from build123d import *

# Parameters (mm, degrees)
CUT_EXTRUDE2_DEPTH = 9.0000094


with BuildPart() as part:
    # Sketch1 → Revolve1 (revolve)
    with BuildSketch(Plane(origin=(0, 0, 0), x_dir=(0, 1, 0), z_dir=(0, 0, 1))):
        with BuildLine():
            Line((4.0000047, 0), (-4.0000047, 0))
            Line((-4.0000047, 0), (-4.0000047, 15.200621907))
            ThreePointArc((-4.0000047, 15.200621907), (-3.862299847, 15.545211447), (-3.525035946, 15.699994))
            ThreePointArc((-3.525035946, 15.699994), (-2.891173009, 15.55542644), (-2.425734949, 15.101499778))
            Line((-2.425734949, 15.101499778), (-1.558842609, 13.5999982))
            ThreePointArc((-1.558842609, 13.5999982), (0, 12.7), (1.558842609, 13.5999982))
            Line((1.558842609, 13.5999982), (2.425734949, 15.101499778))
            ThreePointArc((2.425734949, 15.101499778), (2.891173009, 15.55542644), (3.525035946, 15.699994))
            ThreePointArc((3.525035946, 15.699994), (3.862299847, 15.545211447), (4.0000047, 15.200621907))
            Line((4.0000047, 15.200621907), (4.0000047, 0))
        make_face()
    revolve(axis=Axis((0, 4.0000047, 0), (0, -1, 0)))

    # Sketch2 → Cut-Extrude2 (cut, through all)
    with BuildSketch(Plane.XZ.offset(4.0000047)):
        Polygon((7.332348419, 0), (3.666174209, 6.35), (-3.666174209, 6.35), (-7.332348419, 0), (-3.666174209, -6.35), (3.666174209, -6.35), align=None)
    extrude(amount=-CUT_EXTRUDE2_DEPTH, mode=Mode.SUBTRACT)


solid = part.part
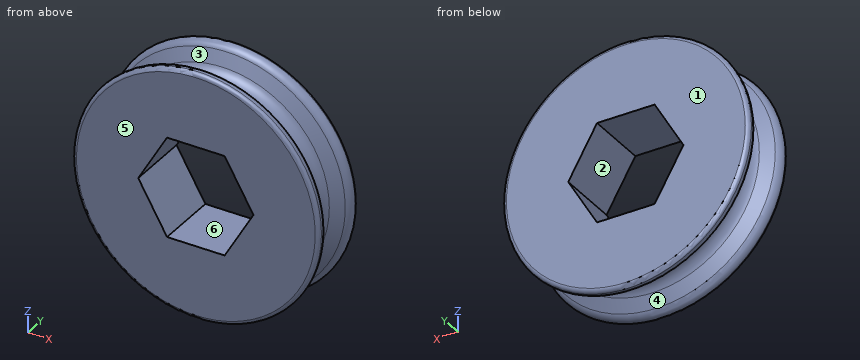
Could you check a few things on this model? Use its own coordinates, in mm. Face numbers are marked on the shaded views. A direction names the side the tool comes from. Coordinates: 2 decimals unless noted, no trailing zeros. Order: outer loops, then holes, each group sorted by start corner. A loop starts at its lowest first (then second) coordinate and runs counter-clockwise, first axis right, second up. Notation, with made-up numbers: (32, 63.25) -> (60, 63.25) arc R10 cw to (60, 82.25) -> close; hole circle Ø8 at (-16, 74). An arc over 180 degrees is marked (long way). One line per item, written item: value. Start each with the question number.
1) If I drill on L1, parallel to X at y = -2.75, z = 0; L2, parallel to Z at x = -1.5, y = 1.75; L3, parallel to Z at x = 6.5, y = -1, over which ranges is the centre line in solid material (lowest first)? Write a range as [from, to].
2) Which directions (+Z, -Z, +X, -X, +Y, -Y) give clear straight access to the entire face, cutting with the end or side of a thin tool? Please do the marked faces 1, 2 and 3.
3) We'd pull the mould along X, two halves only. Please class the marked faces 4, 5 and 6: +X half, -X half, draft (parallel to the pull), parting line (faces both ways), or undercut.
4) I'm going to push flat-ended pins straight in: pin 1 (3 mm diameter, centred on x = -6.5, y = -0.5, fed in from +Z); pin 2 (3 mm diameter, centred on x = 10.5, y = 2, fed in from +Z); pin 3 (1.5 mm diameter, centred on x = 12, y = 2.5, fed in from +Z). Where does each tip first touch, or does it pass through?
5) Imagine slicing it at A-A on x = 0. List the corners of the cut face in (y, z) for me.
Answer list:
1. L1: x = [-15.47, -7.33], [7.33, 15.47]
1. L2: z = [-13.85, -6.35], [6.35, 13.85]
1. L3: z = [-11.26, -1.44], [1.44, 11.26]
2. face 1: +Z, -Z, +X, -X, +Y
2. face 2: +Y, -Y
2. face 3: none
3. face 4: parting line
3. face 5: draft
3. face 6: undercut
4. pin 1: stops at z = 12.9
4. pin 2: stops at z = 12.48
4. pin 3: stops at z = 10.63
5. outline: (-4, -15.2) arc R0.5 ccw to (-3.53, -15.7) arc R1.2 ccw to (-2.43, -15.1) -> (-1.56, -13.6) arc R1.8 cw to (1.56, -13.6) -> (2.43, -15.1) arc R1.2 ccw to (3.53, -15.7) arc R0.5 ccw to (4, -15.2) -> (4, -6.35) -> (-4, -6.35) -> close; (-4, 6.35) -> (4, 6.35) -> (4, 15.2) arc R0.5 ccw to (3.53, 15.7) arc R1.2 ccw to (2.43, 15.1) -> (1.56, 13.6) arc R1.8 cw to (-1.56, 13.6) -> (-2.43, 15.1) arc R1.2 ccw to (-3.53, 15.7) arc R0.5 ccw to (-4, 15.2) -> close
